```python
from build123d import *

# Parameters (mm, degrees)
SKETCH_R          = 6
PAD_DEPTH         = 12
SKETCH001_R       = 2.5
PAD001_DEPTH      = 4
SKETCH002_R       = 13.5
PAD002_DEPTH      = 8.5
SKETCH003_R       = 4
POCKET_DEPTH      = 0.001
POCKET_DEPTH_BACK = 12.001


with BuildPart() as part:
    # Sketch → Pad (new body)
    with BuildSketch(Plane.XY):
        Circle(SKETCH_R)
    extrude(amount=PAD_DEPTH)

    # Sketch001 → Pad001 (join)
    with BuildSketch(Plane.XY):
        with BuildLine():
            ThreePointArc((12.548063, -4.97957), (13.5, 0), (12.548063, 4.97957))
            Line((5, 24), (12.548063, 4.97957))
            Line((-5, 24), (5, 24))
            Line((-5, 24), (-12.548063, 4.97957))
            ThreePointArc((-12.548063, 4.97957), (-13.5, -1.3e-05), (-12.548053, -4.979595))
            Line((-5, -24), (-12.548053, -4.979595))
            Line((-5, -24), (5, -24))
            Line((5, -24), (12.548063, -4.97957))
        make_face()
        with Locations((0, 18)):
            Circle(SKETCH001_R, mode=Mode.SUBTRACT)
        with Locations((0, -18)):
            Circle(SKETCH001_R, mode=Mode.SUBTRACT)
    extrude(amount=PAD001_DEPTH)

    # Sketch002 → Pad002 (join)
    with BuildSketch(Plane.XY):
        Circle(SKETCH002_R)
    extrude(amount=PAD002_DEPTH)

    # Sketch003 → Pocket (cut, two sides)
    with BuildSketch(Plane.XY) as pocket_sk:
        Circle(SKETCH003_R)
    extrude(amount=-POCKET_DEPTH, mode=Mode.SUBTRACT)
    extrude(pocket_sk.sketch, amount=POCKET_DEPTH_BACK, mode=Mode.SUBTRACT)


solid = part.part
```
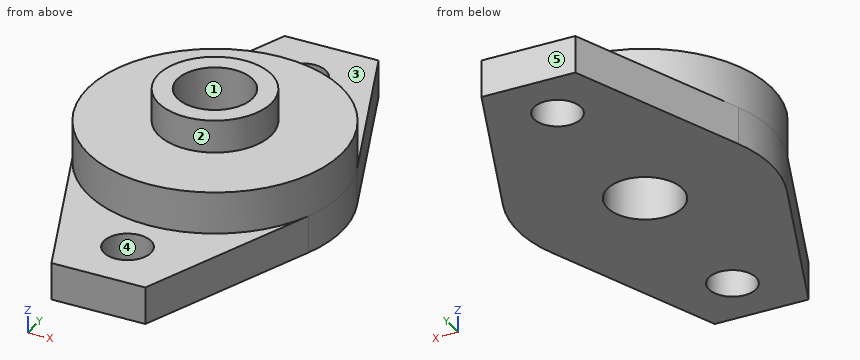
Verification items for the finished model (mm, model axes). Face numbers are marked on the shaded views. A direction names the side the tool comes from. Coordinates: 2 decimals unless noted, no trailing zeros. Loops run counter-clockwise (first coordinate to the right, second up) from the corner with the lowest first, then second, coordinate; pieces in that order, holes last. Notation, with made-up numbers: (76, -12) - (122, -12) arc R18 ccw to (122, -6) - close; hole circle Ø3 at (-4.75, 56.25). An arc over 180 degrees is marked (long way). Answer as a JSON object with one key per item and string values.
(1) Access from +Z, -Z, +X, -X, +Y, -Y to the whole of each face (thin tool, end or side, straight path). Record for the marked faces 1 and 2.
Response:
{"face 1": "+Z, -Z", "face 2": "+Z"}
(2) Cross-section at D-D, the plane x = -4.5. Record the boundary of the cut face in (y, z).
Response:
{"outline": "(-24, 0) - (24, 0) - (24, 4) - (12.73, 4) - (12.73, 8.5) - (3.97, 8.5) - (3.97, 12) - (-3.97, 12) - (-3.97, 8.5) - (-12.73, 8.5) - (-12.73, 4) - (-24, 4) - close"}
(3) Cross-section at B-B, the plane y = 0. Record the boundary of the cut face in (x, z).
Response:
{"outline": "(-13.5, 0) - (-4, 0) - (-4, 12) - (-6, 12) - (-6, 8.5) - (-13.5, 8.5) - close; (4, 0) - (13.5, 0) - (13.5, 8.5) - (6, 8.5) - (6, 12) - (4, 12) - close"}
(4) Cross-section at A-A, the plane x = 0. Record the boundary of the cut face in (y, z), then the cut area to 4 significant figures.
Response:
{"outline": "(-24, 0) - (-20.5, 0) - (-20.5, 4) - (-24, 4) - close; (-15.5, 0) - (-4, 0) - (-4, 12) - (-6, 12) - (-6, 8.5) - (-13.5, 8.5) - (-13.5, 4) - (-15.5, 4) - close; (4, 0) - (15.5, 0) - (15.5, 4) - (13.5, 4) - (13.5, 8.5) - (6, 8.5) - (6, 12) - (4, 12) - close; (20.5, 0) - (24, 0) - (24, 4) - (20.5, 4) - close", "area": "219.5 mm²"}
(5) Go/stop test with flat-tipped pins: pin 1 Ø5 at (x, y) = (9.5, 2) entering from +Z; pin 2 Ø12 at (x, y) = (-10.5, -9) entering from -Z; pin 3 Ø6.5 at (x, y) = (0, 0) entering from -Z. Record where each tip stops, or that it passes through.
Response:
{"pin 1": "stops at z = 8.5", "pin 2": "stops at z = 0", "pin 3": "passes through"}
(6) Cross-section at C-C, the plane z = 6.5. Record the boundary of the cut face in (x, y), then the cut area to 3 significant figures.
Response:
{"outline": "circle Ø27 at (0, 0); hole circle Ø8 at (0, 0)", "area": "522 mm²"}
(7) Mould release check, pull along Y, two halves, no side actions. Record for the marked faces 3, 4 and 5: pulls with the +Y half, pulls with the -Y half, needs draft (parallel to the pull), parting line crosses it, or undercut.
Response:
{"face 3": "needs draft", "face 4": "undercut", "face 5": "pulls with the +Y half"}
(8) Scan lines: line 1 along Y through (x, z) = (0, 1.9); line 2 along Y through (x, z) = (-0.25, 6.75); line 3 along Z through (x, y) = (-6.25, -11.5). Record each from-to range of solid material in increasing order.
Response:
{"line 1": "y = -24 to -20.5, -15.5 to -4, 4 to 15.5, 20.5 to 24", "line 2": "y = -13.5 to -3.99, 3.99 to 13.5", "line 3": "z = 0 to 8.5"}
